The drawing under review shows one solid part. Ordinate dimensions are in mm from its lowest x, y, z. A direction names the side the tool comes from. Coordinates: 2 decimals unless noted, no trailing zeros. Order: outer loops, then holes, each group sorted by start corner. A loop starts at its lowest first (then second) coordinate and runs counter-clockwise, first axis right, second up.
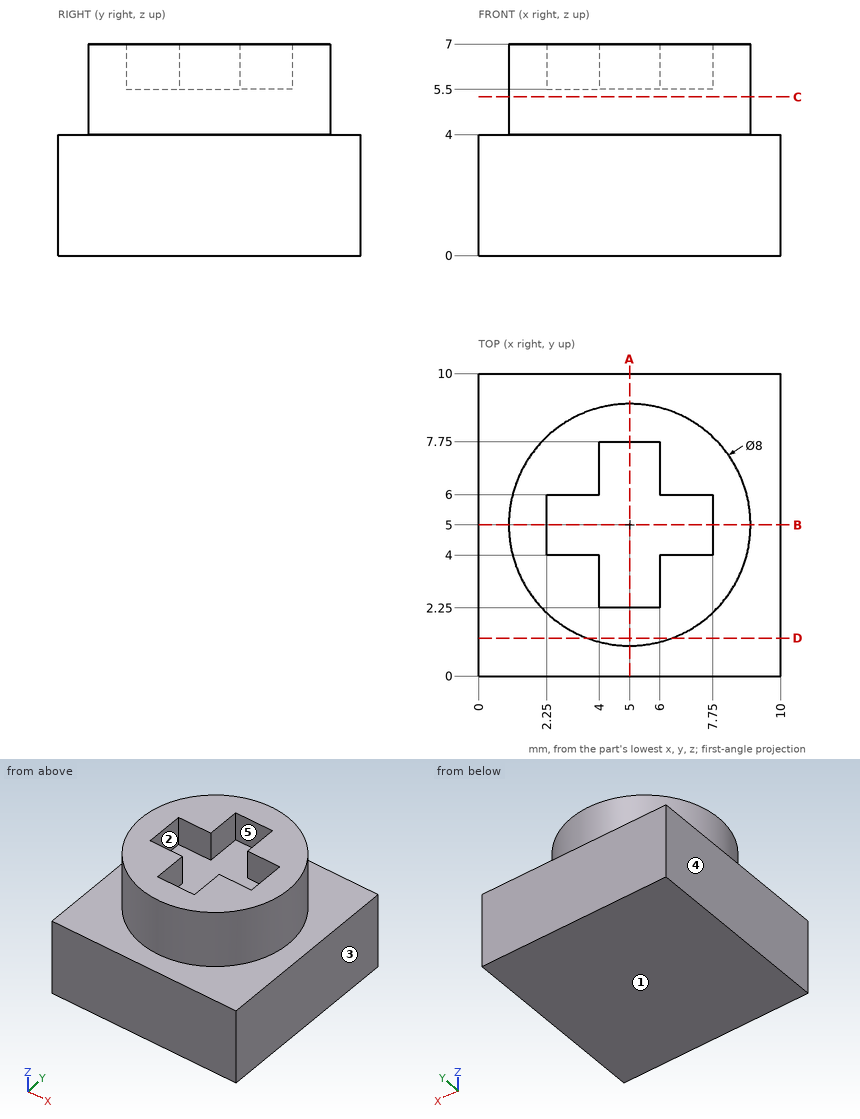
(1) Consider section D-D (y = 1.25). Give the boundary of the cut face in (x, z).
(2) Consider section A-A (x = 5). Give the boundary of the cut face in (y, z).
(3) The part is to be moulded in two halves that separate along X. For the marked faces 1, 2 and 3, say which applies: +X half, -X half, draft (parallel to the pull), parting line (faces both ways), or undercut.
(4) Tool access review of the marked faces 4 and 5: name each direction out of +Z, -Z, +X, -X, +Y, -Y from which nothing blocks a thin tool from reaching the whole face with its end or side.
(5) Insertion check: pin 1 Ø1.6 at (y, z) = (3.5, 6.5) entering from +X; pin 2 Ø1.6 at (x, z) = (2.5, 6.5) entering from -Y; pin 3 Ø1.2 at (y, z) = (5, 6) entering from +X. Each pin has a flat end and moves straight along its axis. Give the tip position at first contact, or say it passes through.
(6) Wall thickness on line 1 (Y direction, x = 3.5, z = 6.75); line 2 (Z direction, x = 1.5, y = 8.5); line 3 (Z direction, x = 4.75, y = 6): over which ranges is each line inside the solid? List them lowest first.
(7) Consider section C-C (z = 5.25). Give the boundary of the cut face in (x, y), then the cut area to 3 significant figures.
Findings:
1. outline: (0, 0) - (10, 0) - (10, 4) - (6.39, 4) - (6.39, 7) - (3.61, 7) - (3.61, 4) - (0, 4) - close
2. outline: (0, 0) - (10, 0) - (10, 4) - (9, 4) - (9, 7) - (7.75, 7) - (7.75, 5.5) - (2.25, 5.5) - (2.25, 7) - (1, 7) - (1, 4) - (0, 4) - close
3. face 1: draft
3. face 2: undercut
3. face 3: +X half
4. face 4: +Z, -Z, -X, +Y, -Y
4. face 5: +Z
5. pin 1: stops at x = 8.94
5. pin 2: stops at y = 1.38
5. pin 3: stops at x = 9
6. line 1: y = 1.29 to 4, 6 to 8.71
6. line 2: z = 0 to 4
6. line 3: z = 0 to 5.5
7. outline: circle Ø8 at (5, 5)
7. area: 50.3 mm2
